Design review of the part built by this model. Coordinates are the model's own, in mm. A direction names the side the tool comes from. Coordinates: 2 decimals unless noted, no trailing zeros. Write each loop counter-clockwise with the first axis right and the second up, starting at its lowest first coordinate (ties: lowest second). Pieces come first, ordered by that corner, then holes. Notation, with made-up numbers: (-35, 77.25) - (-14, 77.25) arc R13 cw to (-14, 86.25) - close; hole circle Ø11 at (35.25, 57). An arc over 180 degrees is marked (long way). Use a Markdown table: item, result.
from build123d import *

# Parameters (mm, degrees)
F1_DEPTH = 3
F2_W     = 12
F2_H     = 6
F3_DEPTH = 23
F4_R     = 2.6556349186
F5_R     = 1.5
F6_DEPTH = 25


with BuildPart() as f1:
    # F0 (on Top) → F1 (new body)
    with BuildSketch(Plane.XY):
        with BuildLine():
            Line((-0.8725353895, 110), (-35.8725353895, 110))
            ThreePointArc((-35.8725353895, 110), (-45.391565001, 87.0190296114), (-68.3725353895, 77.5))
            Line((-68.3725353895, 77.5), (-68.3725353895, 32.5))
            ThreePointArc((-68.3725353895, 32.5), (-45.391565001, 22.9809703886), (-35.8725353895, 0))
            Line((-35.8725353895, 0), (-0.8725353895, 0))
            ThreePointArc((-0.8725353895, 0), (8.6464942219, 22.9809703886), (31.6274646105, 32.5))
            Line((31.6274646105, 32.5), (31.6274646105, 77.5))
            ThreePointArc((31.6274646105, 77.5), (8.6464942219, 87.0190296114), (-0.8725353895, 110))
        make_face()
    extrude(amount=-F1_DEPTH)

    # F2 (on face) → F3 (join)
    with BuildSketch(Plane.XY):
        with Locations((-17.8964557126, 100.6955172337)):
            Rectangle(F2_W, F2_H)
    extrude(amount=F3_DEPTH)

    # F4
    f4_edges = [f1.edges().sort_by_distance(p)[0] for p in [
        (-17.896456, 103.695517, 23),
        (-17.896456, 97.695517, 23),
    ]]
    fillet(f4_edges, radius=F4_R)

    # F5 (on face) → F6 (cut)
    with BuildSketch(Plane.XY):
        with Locations((-9.4853062183, 100.6955172337)):
            Circle(F5_R)
        with Locations((-26.3249855489, 100.6955172337)):
            Circle(F5_R)
        with BuildLine():
            ThreePointArc((-17.9624670977, 91.8832976659), (-16.8593966684, 92.2980970094), (-16.3964557126, 93.381844461))
            ThreePointArc((-16.3964557126, 93.381844461), (-18.9335147568, 94.4655919126), (-17.9624670977, 91.8832976659))
        make_face()
        with BuildLine():
            ThreePointArc((-1.3895297348, 83.3915324938), (-2.8895297348, 84.8915324938), (-4.3895297348, 83.3915324938))
            ThreePointArc((-4.3895297348, 83.3915324938), (-2.8895297348, 81.8915324938), (-1.3895297348, 83.3915324938))
        make_face()
        with BuildLine():
            ThreePointArc((-17.2766075142, 73.4012205266), (-17.6928600626, 74.4382795708), (-18.7105961291, 74.8997673217))
            ThreePointArc((-18.7105961291, 74.8997673217), (-19.8603549658, 72.3641614824), (-17.2766075142, 73.4012205266))
        make_face()
        with Locations((-30.8895297348, 83.3915324938)):
            Circle(F5_R)
        with BuildLine():
            ThreePointArc((22.2231764346, 71.9012205266), (23.2838366064, 72.3405603548), (23.7231764346, 73.4012205266))
            ThreePointArc((23.7231764346, 73.4012205266), (21.1625162629, 74.4618806984), (22.2231764346, 71.9012205266))
        make_face()
        with BuildLine():
            ThreePointArc((23.7231764346, 57.4012205266), (23.2838366064, 58.4618806984), (22.2231764346, 58.9012205266))
            ThreePointArc((22.2231764346, 58.9012205266), (21.1625162629, 56.3405603548), (23.7231764346, 57.4012205266))
        make_face()
        with Locations((-61.5987628698, 73.4012205266)):
            Circle(F5_R)
        with Locations((-61.5987628698, 57.4012205266)):
            Circle(F5_R)
        with Locations((-2.8895297348, 4.9070445821)):
            Circle(F5_R)
        with Locations((-30.8895297348, 4.9070445821)):
            Circle(F5_R)
    extrude(amount=-F6_DEPTH, mode=Mode.SUBTRACT)


solid = f1.part
(1) For pin 1 (1 mm diameter, centred on x = -38.5, y = 75.5, fed in from +Z); pin 2 (6.5 mm diameter, centred on y = 100, z = 16, fed in from -X); pin 3 (6.5 mm diameter, centred on y = 99.5, z = 14.5, fed in from +X), all flat-tipped, find the tip position at first contact; note any pin that passes through.
Determined:
| item | result |
|---|---|
| pin 1 | z = 0 |
| pin 2 | x = -23.9 |
| pin 3 | x = -11.9 |
(2) For L1, parallel to Z at x = -5.5, y = 82; L2, parallel to Y at x = -19, z = 3; L3, parallel to X at y = 7.5, z = -0.75, list the stretches that pass through material, from the lowest coordinate up. Write a range as from..to.
Determined:
| item | result |
|---|---|
| L1 | -3..0 |
| L2 | 97.7..103.7 |
| L3 | -36.75..0 |
(3) Take a section at A-A on y = 52.5. Write out the cut boundary in (x, z), and give its area (3 significant figures).
Determined:
| item | result |
|---|---|
| outline | (-68.37, -3) - (31.63, -3) - (31.63, 0) - (-68.37, 0) - close |
| area | 300 mm2 |
(4) Draft analysis for pull direction X (two halves, no side actions). For faces 4 (the flat face through (-11.896, 101, 11)), 5 (the cylindrical face through (-3.582, 84.722, -1.479)), 6 (the flat face through (-23.896, 101, 11)), state which applies: +X half, -X half, draft (parallel to the pull), parting line (faces both ways), or undercut.
Determined:
| item | result |
|---|---|
| face 4 | +X half |
| face 5 | undercut |
| face 6 | -X half |
(5) Machinability: for faces 1 (the flat face through (-18, 103.696, 10)), 2 (the flat face through (-68.373, 55, -1)), 3 (the flat face through (-18, 97.696, 10)), which of the approach directions +Z, -Z, +X, -X, +Y, -Y give a long, thin tool a straight path to every point of the face, cutting with its end or side? Answer none if there is none.
Determined:
| item | result |
|---|---|
| face 1 | +Z, +X, -X, +Y |
| face 2 | +Z, -Z, -X, +Y, -Y |
| face 3 | +Z, +X, -X, -Y |
(6) Take a section at B-B on x = 4. Write out the cut boundary in (y, z), and give its area (3 significant figures).
Determined:
| item | result |
|---|---|
| outline | (17.12, -3) - (92.88, -3) - (92.88, 0) - (17.12, 0) - close |
| area | 227 mm2 |
